The listing builds one solid part. Answer for the finished solid, in the listing's coordinates (mm). A direction names the side the tool comes from. Give positions to 0.01 mm unless a question says otherwise; leave off trailing zeros. Order: outer loops, then holes, each group sorted by start corner. A loop starts at its lowest first (then second) coordinate and runs counter-clockwise, first axis right, second up. Notation, with made-up numbers: (69, 44.5) - (94, 44.5) arc R25 ccw to (94, 70.5) - close; hole circle Ø4 at (9.25, 63.5). An arc over 180 degrees is marked (long way). Answer as CSV lines item,"result". Start each with the question number.
1. Flat-ended cylindrical pins translate along their axes: pin 1 (1 mm diameter, centred on y = 36.5, z = 2089, fed in from +X); pin 2 (10 mm diameter, centred on x = 976, z = 2303, fed in from +Y); pin 3 (4 mm diameter, centred on x = 255.5, z = 1108.5, fed in from -Y). Find the tip coordinate at first contact, or state that the pin passes through.
2. Which of the six approach directions +Z, -Z, +X, -X, +Y, -Y give full straight-line access (tool end or side, diameter ignored) to faces 1 (the flat face through (419, 16.822, 1296)), 2 (the flat face through (903.45, 33.013, 1296.097)), 3 (the flat face through (280, 51.222, 1296))?
3. Consider line 1 along Y through (x, z) = (455, 2358); line 2 along Y through (x, z) = (343, 744.5). Determine where each line is inside the solid, lowest interval first. Write a range as [from, to].
4. Section A-A on y = 43 is taken. Count the separate pieces of the cut face and the enclosed holes in it, and give its area (3 significant figures).
5. Section B-B on x = 826 is taken. Give the vertices of the cut face in (y, z), and give its area (3 significant figures).
6. Determine the mould class of faces 4 (the flat face through (419, 15.222, 1296)), 5 (the flat face through (697, 16.822, 1296)), 6 (the flat face through (69.45, 33.013, 1296.097)) for opening direction X: +X half, -X half, draft (parallel to the pull), parting line (faces both ways), or undercut.
from build123d import *

# Parameters (mm, degrees)
F1_DEPTH = 2629


with BuildPart() as f1:
    # F0 (on Top) → F1 (new body)
    with BuildSketch(Plane.XY):
        with BuildLine():
            ThreePointArc((103.213446, 15.932448), (104.661294, 15.401879), (106.192738, 15.221745))
            Line((106.192738, 15.221745), (175.807262, 15.221745))
            ThreePointArc((175.807262, 15.221745), (177.338706, 15.401879), (178.786554, 15.932448))
            Line((178.786554, 15.932448), (245.381676, 49.621745))
            Line((245.381676, 49.621745), (314.618324, 49.621745))
            Line((314.618324, 49.621745), (381.213446, 15.932448))
            ThreePointArc((381.213446, 15.932448), (382.661294, 15.401879), (384.192738, 15.221745))
            Line((384.192738, 15.221745), (453.807262, 15.221745))
            ThreePointArc((453.807262, 15.221745), (455.338706, 15.401879), (456.786554, 15.932448))
            Line((456.786554, 15.932448), (523.381676, 49.621745))
            Line((523.381676, 49.621745), (592.618324, 49.621745))
            Line((592.618324, 49.621745), (659.213446, 15.932448))
            ThreePointArc((659.213446, 15.932448), (660.661294, 15.401879), (662.192738, 15.221745))
            Line((662.192738, 15.221745), (731.807262, 15.221745))
            ThreePointArc((731.807262, 15.221745), (733.338706, 15.401879), (734.786554, 15.932448))
            Line((734.786554, 15.932448), (801.381676, 49.621745))
            Line((801.381676, 49.621745), (870.618324, 49.621745))
            Line((870.618324, 49.621745), (937.213446, 15.932448))
            ThreePointArc((937.213446, 15.932448), (938.661294, 15.401879), (940.192738, 15.221745))
            Line((940.192738, 15.221745), (1009.807262, 15.221745))
            ThreePointArc((1009.807262, 15.221745), (1011.338706, 15.401879), (1012.786554, 15.932448))
            Line((1012.786554, 15.932448), (1079.381676, 49.621745))
            Line((1079.381676, 49.621745), (1116, 49.621745))
            Line((1116, 49.621745), (1116, 51.221745))
            Line((1116, 51.221745), (1080.192738, 51.221745))
            ThreePointArc((1080.192738, 51.221745), (1079.032553, 51.08528), (1077.935699, 50.683334))
            Line((1077.935699, 50.683334), (1012.064301, 17.360156))
            ThreePointArc((1012.064301, 17.360156), (1010.967447, 16.95821), (1009.807262, 16.821745))
            Line((1009.807262, 16.821745), (940.192738, 16.821745))
            ThreePointArc((940.192738, 16.821745), (939.032553, 16.95821), (937.935699, 17.360156))
            Line((937.935699, 17.360156), (872.064301, 50.683334))
            ThreePointArc((872.064301, 50.683334), (870.967447, 51.08528), (869.807262, 51.221745))
            Line((869.807262, 51.221745), (802.192738, 51.221745))
            ThreePointArc((802.192738, 51.221745), (801.032553, 51.08528), (799.935699, 50.683334))
            Line((799.935699, 50.683334), (734.064301, 17.360156))
            ThreePointArc((734.064301, 17.360156), (732.967447, 16.95821), (731.807262, 16.821745))
            Line((731.807262, 16.821745), (662.192738, 16.821745))
            ThreePointArc((662.192738, 16.821745), (661.032553, 16.95821), (659.935699, 17.360156))
            Line((659.935699, 17.360156), (594.064301, 50.683334))
            ThreePointArc((594.064301, 50.683334), (592.967447, 51.08528), (591.807262, 51.221745))
            Line((591.807262, 51.221745), (524.192738, 51.221745))
            ThreePointArc((524.192738, 51.221745), (523.032553, 51.08528), (521.935699, 50.683334))
            Line((521.935699, 50.683334), (456.064301, 17.360156))
            ThreePointArc((456.064301, 17.360156), (454.967447, 16.95821), (453.807262, 16.821745))
            Line((453.807262, 16.821745), (384.192738, 16.821745))
            ThreePointArc((384.192738, 16.821745), (383.032553, 16.95821), (381.935699, 17.360156))
            Line((381.935699, 17.360156), (316.064301, 50.683334))
            ThreePointArc((316.064301, 50.683334), (314.967447, 51.08528), (313.807262, 51.221745))
            Line((313.807262, 51.221745), (246.192738, 51.221745))
            ThreePointArc((246.192738, 51.221745), (245.032553, 51.08528), (243.935699, 50.683334))
            Line((243.935699, 50.683334), (178.064301, 17.360156))
            ThreePointArc((178.064301, 17.360156), (176.967447, 16.95821), (175.807262, 16.821745))
            Line((175.807262, 16.821745), (106.192738, 16.821745))
            ThreePointArc((106.192738, 16.821745), (105.032553, 16.95821), (103.935699, 17.360156))
            Line((103.935699, 17.360156), (38.064301, 50.683334))
            ThreePointArc((38.064301, 50.683334), (36.967447, 51.08528), (35.807262, 51.221745))
            Line((35.807262, 51.221745), (0, 51.221745))
            Line((0, 51.221745), (0, 49.621745))
            Line((0, 49.621745), (36.618324, 49.621745))
            Line((36.618324, 49.621745), (103.213446, 15.932448))
        make_face()
    extrude(amount=F1_DEPTH)


solid = f1.part
Checks:
1,pin 1,"stops at x = 1054.43"
1,pin 2,"stops at y = 16.82"
1,pin 3,"stops at y = 49.62"
2,face 1,"+Z, -Z, +Y"
2,face 2,"+Z, -Z, -Y"
2,face 3,"+Z, -Z, +X, -X, +Y"
3,line 1,"y = [15.33, 16.97]"
3,line 2,"y = [35.26, 37.06]"
4,separate pieces,"8"
4,enclosed holes,"0"
4,area,"74,500 mm²"
5,outline,"(49.62, 0) - (51.22, 0) - (51.22, 2629) - (49.62, 2629) - close"
5,area,"4,210 mm²"
6,face 4,"draft"
6,face 5,"undercut"
6,face 6,"-X half"
